Answer from the drawing. Dimensions are ordinates in mm from the lowest x, y and z of the part. Round coordinates to 2 decimals unless told otherwise and drop trailing zeros. Loops run counter-clockwise (first coordinate to the right, second up) from the corner with the lowest first, then second, coordinate; pieces in that order, holes last. Notation, with made-up numbers: M 73,-15.75 L 112,-15.75 A26 ccw 112,21.25 Z; hole C 28.25,37.25 d9. An arc over 180 degrees is marked long. One line per item, written item: value.
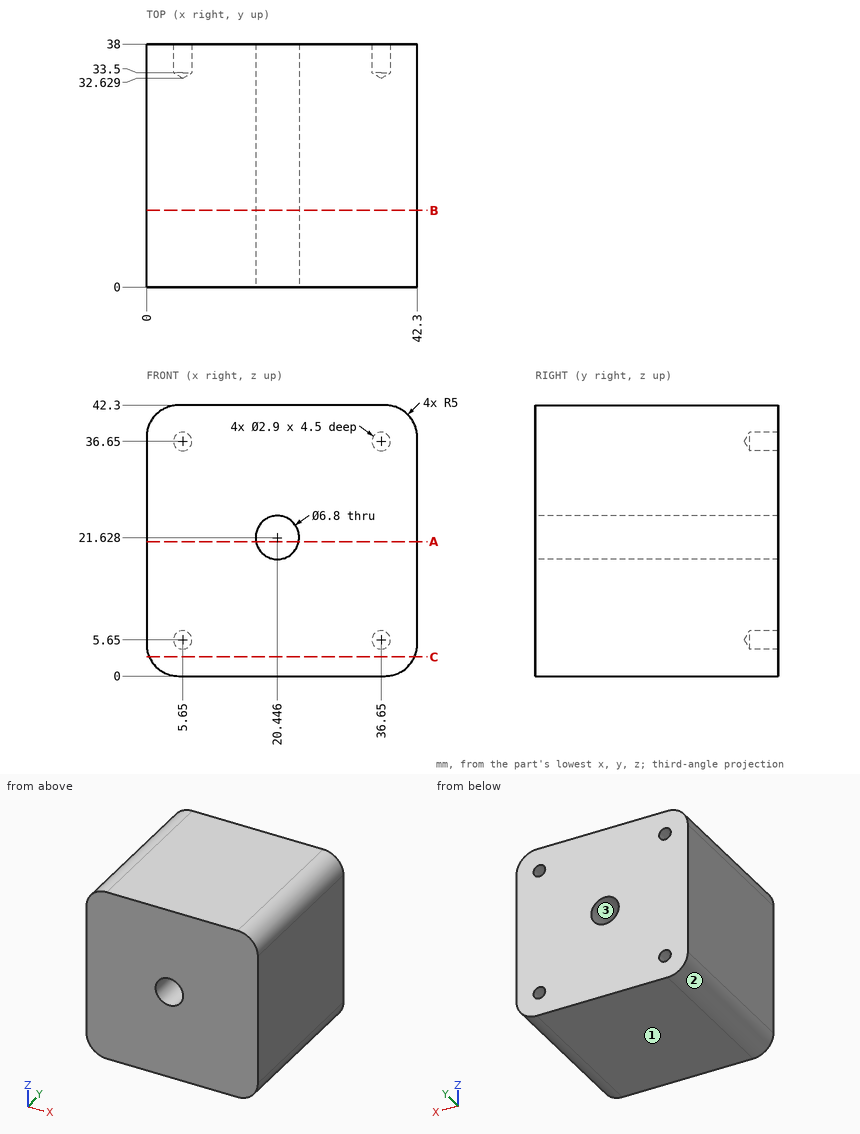
1) Find the intervals of material crossed by probe 1 along X at (y, z) = (36.8, 36.65); probe 2 along Z at (x, y) = (5, 36); probe 3 along X at (y, z) = (11.5, 37.5), in increasing order. Write a range as from..to.
Check values:
probe 1: 0..4.2, 7.1..35.2, 38.1..42.3
probe 2: 0..4.35, 6.95..35.35, 37.95..42.3
probe 3: 0..42.3
2) Find section B-B (y = 12). Give the vertices of the cut face in (x, z), then the cut area to 3 significant figures.
Check values:
outline: M 0,5 A5 ccw 5,0 L 37.3,0 A5 ccw 42.3,5 L 42.3,37.3 A5 ccw 37.3,42.3 L 5,42.3 A5 ccw 0,37.3 Z; hole C 20.45,21.63 d6.8
area: 1,730 mm2
3) Find section A-A (z = 21). Give the vertices of the cut face in (x, y) (1 decimal), then the cut area to 3 significant figures.
Check values:
outline: M 0,0 L 17.1,0 L 17.1,38 L 0,38 Z; M 23.8,0 L 42.3,0 L 42.3,38 L 23.8,38 Z
area: 1,350 mm2
4) The mould has two halves that part along X. Classify the marked faces 1, 2 and 3: +X half, -X half, draft (parallel to the pull), parting line (faces both ways), or undercut.
Check values:
face 1: draft
face 2: -X half
face 3: undercut
5) Find section C-C (z = 3). Give the vertices of the cut face in (x, y), then the cut area to 3 significant figures.
Check values:
outline: M 0.42,0 L 41.88,0 L 41.88,38 L 0.42,38 Z
area: 1,580 mm2
